Work out the finished part from the listing and answer in its coordinate system (mm). A direction names the side the tool comes from. Round coordinates to 2 decimals unless told otherwise and drop trailing zeros. Loops run counter-clockwise (first coordinate to the right, second up) from the corner with the lowest first, then second, coordinate; pieces in that order, holes last. Notation, with made-up numbers: (12.25, 85.5) - (18.25, 85.5) arc R11 cw to (18.25, 92.5) - close; hole circle Ø9 at (81, 53.25). An arc over 180 degrees is marked (long way). Answer as CSV lines item,"result". Start each with the question number.
Q1. For faces 4 (the face through (-0.52, 23.55, -6.36)), 5 (the face through (121.97, 6.08, -0.62)), determine the directions among +Z, -Z, +X, -X, +Y, -Y from which every point of the face is accessible in a straight line to the end or side of a thin tool.
Q2. Straight lines are drawn through the part: L1, parallel to Z at x = 0, y = 3; L2, parallel to X at y = 13.5, z = -0.25; L3, parallel to X at y = 7.5, z = -1.25. For each, find the intervals that lie inside material, in ascending order. Write a range as [from, to].
Q3. Section A-A on y = 10.5 is taken. Write down the section's boundary in (x, z), then the cut area to 3 significant figures.
Q4. Section B-B on x = 105.5 is taken. Write down the section's boundary in (y, z), then the cut area to 3 significant figures.
Q5. Each of these flat-tipped pins is pushed along its axis until it touches: pin 1 Ø8 at (x, z) = (90, -4.5) entering from +Y; pin 2 Ø3 at (x, z) = (95.5, -7) entering from -Y; pin 3 Ø2.5 at (x, z) = (120, 0) entering from -Y. Where does it stop, or does it pass through?
Q6. The mould has two halves that part along Z. Classify faces 1 (the face through (120.4, 13, 0)), 2 (the face through (61, 40, -10)), 3 (the face through (-2, 0, 2)): +Z half, -Z half, draft (parallel to the pull), parting line (faces both ways), or undercut.
```python
from build123d import *

# Parameters (mm, degrees)
SKETCH2_R  = 4
TAP1_D     = 4.134
TAP1_DEPTH = 12
TAP1_TIP   = 1.2419789


with BuildPart() as part:
    # Sweep1: sweep along a curve in space
    with BuildLine() as sweep1_path:
        Line((0, 0, 0), (0, 18.16, 0))
        ThreePointArc((0, 18.16, 0), (0, 21.091478934, -0.439328933), (0, 23.765381166, -1.718713748))
        Line((0, 23.765381166, -1.718713748), (0, 27.718713748, -4.394618834))
        ThreePointArc((0, 27.718713748, -4.394618834), (2.928932188, 33.574467414, -8.358221868), (10, 36, -10))
        Line((10, 36, -10), (110, 36, -10))
        ThreePointArc((120, 27.718713748, -4.394618834), (117.071067812, 33.574467414, -8.358221868), (110, 36, -10))
        Line((120, 27.718713748, -4.394618834), (120, 23.765381166, -1.718713748))
        ThreePointArc((120, 18.16, 0), (120, 21.091478934, -0.439328933), (120, 23.765381166, -1.718713748))
        Line((120, 18.16, 0), (120, 0, 0))
    # Sketch2 → Sweep1 (sweep)
    with BuildSketch(Plane(origin=(0, 0, 0), x_dir=(1, 0, 0), z_dir=(0, 1, 0))):
        Circle(SKETCH2_R)
    sweep(path=sweep1_path.line)

    # Tap1
    with Locations(Plane(origin=(0, 0, 0), x_dir=(-1, 0, 0), z_dir=(0, -1, 0))):
        with Locations((0, 0), (-120, 0)):
            Hole(TAP1_D / 2, depth=TAP1_DEPTH)
            with Locations((0, 0, -(TAP1_DEPTH + TAP1_TIP / 2))):  # 118° drill point
                Cone(0, TAP1_D / 2, TAP1_TIP, mode=Mode.SUBTRACT)


solid = part.part
```
Findings:
1,face 4,"none"
1,face 5,"-Y"
2,L1,"z = [-4, -2.07], [2.07, 4]"
2,L2,"x = [-3.99, 3.99], [116.01, 123.99]"
2,L3,"x = [-3.8, -1.65], [1.65, 3.8], [116.2, 118.35], [121.65, 123.8]"
3,outline,"circle Ø8 at (0, 0); circle Ø8 at (120, 0); hole circle Ø4.13 at (0, 0); hole circle Ø4.13 at (120, 0)"
3,area,"73.7 mm^2"
4,outline,"circle Ø8 at (36, -10)"
4,area,"50.3 mm^2"
5,pin 1,"stops at y = 39.71"
5,pin 2,"stops at y = 32.29"
5,pin 3,"stops at y = 12.49"
6,face 1,"undercut"
6,face 2,"parting line"
6,face 3,"draft"
